Design review of the part shown in the three views and the two pictorial views. Dimensions are in mm from the part's minimum x, y and z. A direction names the side the tool comes from. Give positions to 0.01 mm unless a question says otherwise; leave off trailing zeros. Loops run counter-clockwise (first coordinate to the right, second up) from the corner with the lowest first, then second, coordinate; pieces in that order, holes last. Notation, with made-up numbers: (3, -27.5) - (33, -27.5) arc R20 cw to (33, -14.5) - close; hole circle Ø5 at (78, 13.25). An arc over 180 degrees is marked (long way). Answer as a JSON object with one key per item and string values.
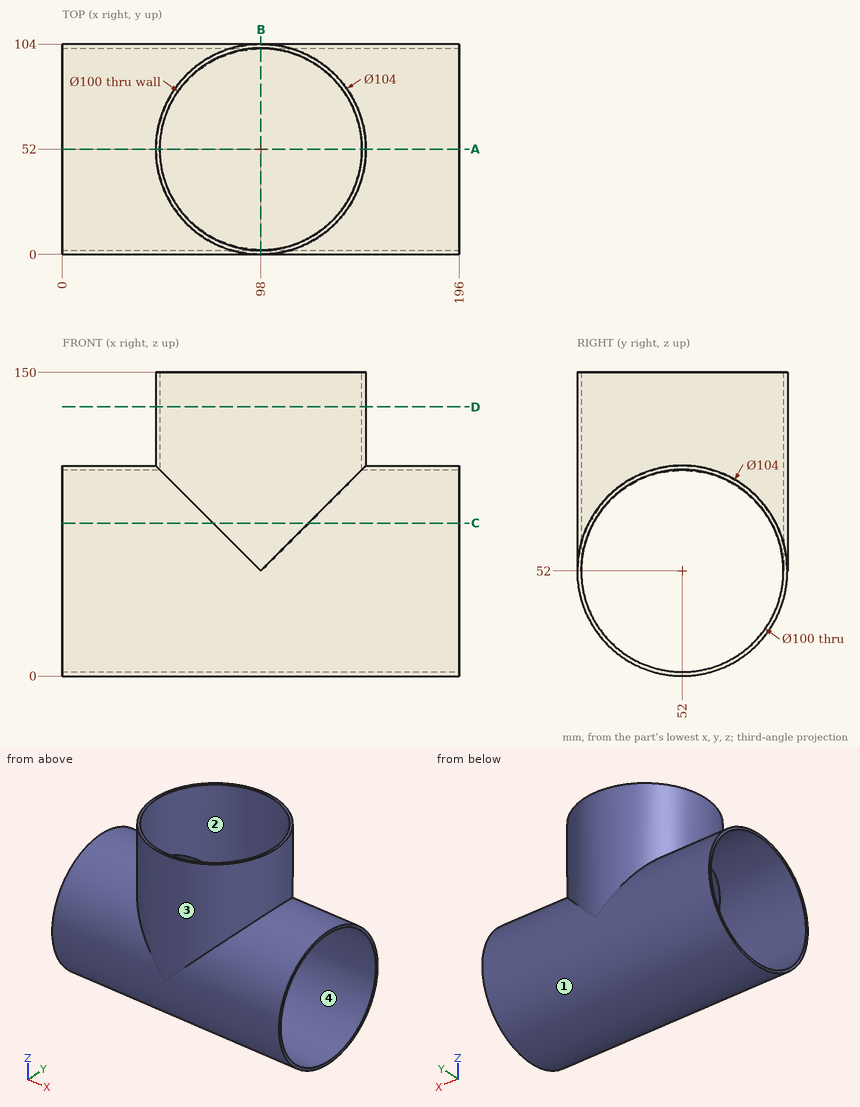
Q1. Consider section C-C, the plane z = 75.5. State the section outline as (x, y) points.
Results:
{"outline": "(0, 5.61) - (74.5, 5.61) arc R52 ccw to (121.5, 5.61) - (196, 5.61) - (196, 7.87) - (121.5, 7.87) arc R50 cw to (74.5, 7.87) - (0, 7.87) - close; (0, 96.13) - (74.5, 96.13) arc R50 cw to (121.5, 96.13) - (196, 96.13) - (196, 98.39) - (121.5, 98.39) arc R52 ccw to (74.5, 98.39) - (0, 98.39) - close"}
Q2. Consider section D-D, the plane z = 133. State the section outline as (x, y) points.
Results:
{"outline": "circle Ø104 at (98, 52); hole circle Ø100 at (98, 52)"}
Q3. Consider section A-A, the plane y = 52. State the section outline as (x, z) points.
Results:
{"outline": "(0, 0) - (196, 0) - (196, 2) - (0, 2) - close; (0, 102) - (48, 102) - (48, 150) - (46, 150) - (46, 104) - (0, 104) - close; (148, 102) - (196, 102) - (196, 104) - (150, 104) - (150, 150) - (148, 150) - close"}
Q4. To check wall thickness, follow probe 1 along Y at (x, z) = (98, 119); probe 2 along X at (y, z) = (52, 114.5); probe 3 along Z at (x, y) = (33.5, 53). State the ranges of each line that lie inside material, in increasing order. Write a range as [from, to].
Results:
{"probe 1": "y = [0, 2], [102, 104]", "probe 2": "x = [46, 48], [148, 150]", "probe 3": "z = [0.01, 2.01], [101.99, 103.99]"}
Q5. For the marked faces 3 and 4, list the 3-axis set-ups (+Z, -Z, +X, -X, +Y, -Y) from which the entire face can be reached by the end or side of a thin tool; tool diameter is ignored.
Results:
{"face 3": "+Z", "face 4": "+X, -X"}
Q6. Consider section B-B, the plane x = 98. State the section outline as (y, z) points.
Results:
{"outline": "(0, 52) arc R52 ccw to (104, 52) - (104, 150) - (102, 150) - (102, 52) arc R50 cw to (2, 52) - (2, 150) - (0, 150) - close"}
Q7. The part is to be moulded in two halves that separate along Y. For the marked faces 1 and 2, say which applies: +Y half, -Y half, draft (parallel to the pull), parting line (faces both ways), or undercut.
Results:
{"face 1": "parting line", "face 2": "undercut"}
Q8. Clearance check with flat-ended pins moving along their axes: pin 1 Ø2 at (x, z) = (51, 62) entering from -Y; pin 2 Ø8 at (x, z) = (139, 129) entering from +Y; pin 3 Ø5 at (x, y) = (62.5, 16.5) entering from -Z. State where each tip first meets the part, or that it passes through.
Results:
{"pin 1": "stops at y = 0.78", "pin 2": "stops at y = 88.54", "pin 3": "stops at z = 11.81"}
